```python
from build123d import *

# Parameters (mm, degrees)
F0_W     = 152.4
F0_H     = 76.2
F1_DEPTH = 76.2
F2_W     = 136.779776
F2_H     = 65.982648
F3_DEPTH = 50.8
F5_DEPTH = 12.7
F7_DEPTH = 12.7
F8_R     = 25.4
F9_DEPTH = 66.04


with BuildPart() as f1:
    # F0 (on Front) → F1 (new body)
    with BuildSketch(Plane.XZ):
        with Locations((-16.745566, 0.768143)):
            Rectangle(F0_W, F0_H)
    extrude(amount=F1_DEPTH)

    # F2 (on face) → F3 (cut)
    with BuildSketch(Plane.XY.offset(38.868143)):
        with Locations((-16.745566, -38.1)):
            Rectangle(F2_W, F2_H)
    extrude(amount=-F3_DEPTH, mode=Mode.SUBTRACT)

    # F4 (on face) → F5 (join)
    with BuildSketch(Plane.YZ.offset(-85.135454)):
        with BuildLine():
            ThreePointArc((-25.4, 38.868143), (-38.1, 26.168143), (-50.8, 38.868143))
            Line((-50.8, 38.868143), (-63.5, 38.868143))
            Line((-63.5, 38.868143), (-63.5, -11.931857))
            Line((-63.5, -11.931857), (-12.7, -11.931857))
            Line((-12.7, -11.931857), (-12.7, 38.868143))
            Line((-12.7, 38.868143), (-25.4, 38.868143))
        make_face()
    extrude(amount=F5_DEPTH)

    # F6 (on face) → F7 (join)
    with BuildSketch(Plane(origin=(51.644322, 0, 0), x_dir=(0, -1, 0), z_dir=(-1, 0, 0))):
        with BuildLine():
            ThreePointArc((50.8, 38.868143), (38.1, 26.168143), (25.4, 38.868143))
            Line((25.4, 38.868143), (12.7, 38.868143))
            Line((12.7, 38.868143), (12.7, -11.931857))
            Line((12.7, -11.931857), (63.5, -11.931857))
            Line((63.5, -11.931857), (63.5, 38.868143))
            Line((63.5, 38.868143), (50.8, 38.868143))
        make_face()
    extrude(amount=F7_DEPTH)

    # F8 (on face) → F9 (cut)
    with BuildSketch(Plane.XY.offset(-11.931857)):
        with Locations((-16.745566, -38.1)):
            Circle(F8_R)
    extrude(amount=-F9_DEPTH, mode=Mode.SUBTRACT)


solid = f1.part
```
Can you work these out from the model? Positions are in its coordinate system, mm. A direction names the side the tool comes from. Round coordinates to 2 decimals unless told otherwise and drop trailing zeros. Order: outer loops, then holes, each group sorted by start corner. A loop starts at its lowest first (then second) coordinate and runs counter-clockwise, first axis right, second up. Notation, with made-up numbers: (-12, -20) -> (43, -20) arc R22 cw to (43, 4) -> close; hole circle Ø6 at (10.5, -12.75). An arc over 180 degrees is marked (long way). Return JSON: item names as keys, results as strings. Group by question number.
1. If we section it at A-A, the plane y = -38.1: Write out the boundary of the cut face in (x, z).
2. I need wall thicknesses on line 1 (Y direction, x = 40, z = -7); line 2 (Y direction, x = -19, z = 12); line 3 (X direction, y = -38, z = -23). Which ranges of each line are inside material? Lowest first, please. Write a range as [from, to].
3. If we section it at B-B, the plane z = 11.5: Write out the boundary of the cut face in (x, y).
4. Which directions (+Z, -Z, +X, -X, +Y, -Y) give clear straight access to the entire face, cutting with the end or side of a thin tool? Please do faces 1 (the face through (-20.052, -12.916, -24.454)), 2 (the face through (-72.435, -38, 14)).
5. If we section it at C-C, the plane x = -44: Write out the boundary of the cut face in (y, z), then the cut area to 3 significant figures.
6. If we section it at D-D, the plane x = -1: Write out the boundary of the cut face in (y, z).
7. We'd pull the mould along Y, two halves only. Please class faces 3 (the face through (-18, -12, -37.332)), 4 (the face through (-18, 0, 1)), 5 (the face through (-18, -5.109, 14)): released by +Y, released by -Y, zero draft, split by the parting line, or undercut.
Output values:
{
 "1": {"outline": "(-92.95, -37.33) -> (-42.15, -37.33) -> (-42.15, -11.93) -> (-72.44, -11.93) -> (-72.44, 26.17) -> (-85.14, 26.17) -> (-85.14, 38.87) -> (-92.95, 38.87) -> close; (8.65, -37.33) -> (59.45, -37.33) -> (59.45, 38.87) -> (51.64, 38.87) -> (51.64, 26.17) -> (38.94, 26.17) -> (38.94, -11.93) -> (8.65, -11.93) -> close"},
 "2": {"line 1": "[-76.2, -71.09], [-63.5, -12.7], [-5.11, 0]", "line 2": "[-76.2, -71.09], [-5.11, 0]", "line 3": "[-92.95, -42.15], [8.65, 59.45]"},
 "3": {"outline": "(-92.95, -76.2) -> (59.45, -76.2) -> (59.45, 0) -> (-92.95, 0) -> close; hole (-85.14, -71.09) -> (51.64, -71.09) -> (51.64, -63.5) -> (38.94, -63.5) -> (38.94, -12.7) -> (51.64, -12.7) -> (51.64, -5.11) -> (-85.14, -5.11) -> (-85.14, -12.7) -> (-72.44, -12.7) -> (-72.44, -63.5) -> (-85.14, -63.5) -> close"},
 "4": {"face 1": "+Z, -Z", "face 2": "+Z"},
 "5": {"outline": "(-76.2, -37.33) -> (0, -37.33) -> (0, 38.87) -> (-5.11, 38.87) -> (-5.11, -11.93) -> (-71.09, -11.93) -> (-71.09, 38.87) -> (-76.2, 38.87) -> close", "area": "2,450 mm²"},
 "6": {"outline": "(-76.2, -37.33) -> (-58.03, -37.33) -> (-58.03, -11.93) -> (-71.09, -11.93) -> (-71.09, 38.87) -> (-76.2, 38.87) -> close; (-18.17, -37.33) -> (0, -37.33) -> (0, 38.87) -> (-5.11, 38.87) -> (-5.11, -11.93) -> (-18.17, -11.93) -> close"},
 "7": {"face 3": "zero draft", "face 4": "released by +Y", "face 5": "undercut"}
}
